Verification items for the finished model (mm, model axes). A direction names the side the tool comes from. Round coordinates to 2 decimals unless told otherwise and drop trailing zeros. Write each loop counter-clockwise with the first axis right and the second up, starting at its lowest first coordinate (ties: lowest second). Pieces come first, ordered by that corner, then holes. Notation, with made-up numbers: M -19,35.25 L 40,35.25 A21 cw 40,43.25 Z; hole C -6.75,-21.5 d2. An arc over 180 degrees is marked long. Write each question's results on one line, items separated by ' | '.
Autodesk Inventor part; units mm, degrees
ref_plane "YZ Plane" through (0, 0, 0) normal (1, 0, 0) x (0, 1, 0)
ref_plane "XZ Plane" through (0, 0, 0) normal (0, 1, 0) x (-1, 0, 0)
ref_plane "XY Plane" through (0, 0, 0) normal (0, 0, 1) x (1, 0, 0)
sketch "Sketch1" plane through (0, 0, 0) normal (0, 1, 0) x (-1, 0, 0)
  line L0 (0, 0) -> (25.4, 0)
  line L1 (25.4, 0) -> (25.4, -25.4)
  line L2 (25.4, -25.4) -> (0, -25.4)
  line L3 (0, -25.4) -> (0, 0)
  line L4 (3.175, -3.175) -> (22.225, -3.175)
  line L5 (22.225, -3.175) -> (22.225, -22.225)
  line L6 (22.225, -22.225) -> (3.175, -22.225)
  line L7 (3.175, -22.225) -> (3.175, -3.175)
  dimension "d0" = 25.4
  dimension "d1" = 25.4
  dimension "d2" = 19.05
  dimension "d3" = 19.05
  dimension "d4" = 3.175
  dimension "d5" = 3.175
extrude "Extrusion1" add sketch "Sketch1" along normal blind 1012.825
sketch "Sketch2" plane through (-25.4, 0, -25.4) normal (-1, 0, 0) x (0, 0, 1)
  line L0 (25.4, 0) -> (0, 0)
  line L1 (25.4, 0) -> (25.4, 1012.825)
  line L2 (0, 1012.825) -> (25.4, 1012.825)
  line L3 (0, 0) -> (0, 1012.825)
  point P0 (12.7, 12.7)
  point P1 (12.7, 38.1)
  dimension "d8" = 12.7
  dimension "d9" = 38.1
  dimension "d14" = 12.7
  dimension "d15" = 12.7
hole "Hole1" at (-25.4, 12.7, -12.7) at (-25.4, 38.1, -12.7) direction (1, 0, 0) diameter 6.35 end through all
sketch "Sketch3" plane through (-25.4, 0, -25.4) normal (-1, 0, 0) x (0, 0, 1)
  circle A0 centre (12.7, 12.7) radius 3.175
  circle A1 centre (12.7, 38.1) radius 3.175
  line L0 (25.4, 0) -> (0, 0)
  line L1 (25.4, 0) -> (25.4, 1012.825)
  line L2 (0, 1012.825) -> (25.4, 1012.825)
  line L3 (0, 0) -> (0, 1012.825)
  line L4 (25.4, 1012.825) -> (0, 1012.825)
  line L5 (0, 1012.825) -> (0, 968.8309)
  line L6 (0, 0) -> (0, 1012.825)
  line L7 (0, 968.8309) -> (25.4, 1012.825)
  dimension "d57" = 60
extrude "Extrusion2" cut sketch "Sketch3" against normal blind 25.4 contours L7 L3 L2
sketch "Sketch5" plane through (-25.4, 0, -25.4) normal (-1, 0, 0) x (0, 0, 1)
  line L0 (25.4, 0) -> (0, 0)
  line L1 (25.4, 0) -> (25.4, 1012.825)
  point P0 (12.7, 774.7)
  dimension "d58" = 12.7
  dimension "d59" = 774.7
hole "Hole5" at (-25.4, 774.7, -12.7) direction (1, 0, 0) diameter 6.35 end through all
sketch "Sketch6" plane through (-25.4, 0, -25.4) normal (-1, 0, 0) x (0, 0, 1)
  line L0 (0, 0) -> (0, 968.8309)
  line L1 (25.4, 0) -> (0, 0)
  point P0 (12.7, 939.8)
  point P1 (12.7, 863.6)
  dimension "d67" = 12.7
  dimension "d68" = 12.7
  dimension "d69" = 863.6
  dimension "d70" = 939.8
hole "Hole6" at (-25.4, 939.8, -12.7) at (-25.4, 863.6, -12.7) direction (1, 0, 0) diameter 6.35 end through all
sketch "Sketch10" plane through (-25.4, 0, 0) normal (0, 0, 1) x (1, 0, 0)
  line L0 (25.4, 0) -> (0, 0)
  line L1 (0, 0) -> (0, 1012.825)
  point P0 (12.7, 628.65)
  point P1 (12.7, 571.5)
  point P2 (12.7, 520.7)
  point P3 (12.7, 889)
  point P4 (12.7, 831.85)
  point P5 (12.7, 177.8)
  dimension "d114" = 12.7
  dimension "d115" = 12.7
  dimension "d116" = 889
  dimension "d117" = 831.85
  dimension "d118" = 571.5
  dimension "d119" = 628.65
  dimension "d120" = 12.7
  dimension "d121" = 12.7
  dimension "d122" = 12.7
  dimension "d123" = 520.7
  dimension "d124" = 177.8
  dimension "d125" = 12.7
hole "Hole10" at (-12.7, 628.65, 0) at (-12.7, 571.5, 0) at (-12.7, 520.7, 0) at (-12.7, 889, 0) at (-12.7, 831.85, 0) at (-12.7, 177.8, 0) direction (0, 0, -1) diameter 6.35 end through all
sketch "Sketch11" plane through (-25.4, 0, -25.4) normal (-1, 0, 0) x (0, 0, 1)
  circle A0 centre (12.7, 939.8) radius 3.175
  circle A1 centre (12.7, 863.6) radius 3.175
  circle A2 centre (12.7, 774.7) radius 3.175
  line L0 (25.4, 1012.825) -> (0, 968.8309)
  line L1 (0, 0) -> (0, 968.8309)
  line L2 (25.4, 0) -> (0, 0)
  line L3 (25.4, 0) -> (25.4, 1012.825)
  circle A3 centre (12.7, 38.1) radius 3.175
  circle A4 centre (12.7, 12.7) radius 3.175
  point P0 (12.7, 57.15)
  dimension "d133" = 57.15
  dimension "d134" = 12.7
hole "Hole11" at (-25.4, 57.15, -12.7) direction (1, 0, 0) diameter 6.35 end through all
properties part number "1x1 support" material "Aluminum 6061"
1) Material ranges on line 1 (X direction, y = 49.5, z = -8.25) (3 decimals); line 2 (X direction, y = 889, z = -24.65) (3 decimals), recorded low to high. Write a range as [from, to].
Calculated:
line 1: x = [-25.4, -22.225], [-3.175, 0] | line 2: x = [-25.4, -15.875], [-9.525, 0]
2) Depth check by flat-ended pin: P1, Ø1, axis at x = -3.5, z = -16.5, coming from the -Y side. Enter the tip coordinate at first touch or a pass-through.
Calculated:
P1: stops at y = 0
3) Draft check along X on faces 3 (the flat face through (-25.4, 499, -13)), 4 (the flat face through (-13, 478, -25.4)), 5 (the flat face through (-22.225, 497, -13)). Enter one of: pulls with the +X half, pulls with the -X half, needs draft (parallel to the pull), parting line crosses it, or undercut.
Calculated:
face 3: pulls with the -X half | face 4: needs draft | face 5: undercut
4) Sectioned sample at A-A, the plane y = 319. Record the cut outline in (x, z) (3 decimals), and give its area (3 significant figures).
Calculated:
outline: M -25.4,-25.4 L 0,-25.4 L 0,0 L -25.4,0 Z; hole M -22.225,-22.225 L -3.175,-22.225 L -3.175,-3.175 L -22.225,-3.175 Z | area: 282 mm²
5) Access from +Z, -Z, +X, -X, +Y, -Y to the whole of each face (thin tool, end or side, straight path). Record for faces 1 (the flat face through (-13, 499, 0)), 2 (the flat face through (-3.175, 497, -13)).
Calculated:
face 1: +Z, +X, -X, +Y, -Y | face 2: +Y, -Y
